from build123d import *

# Parameters (mm, degrees)
F0_W     = 304.8
F0_H     = 297.18
F0_H_2   = 20.32
F1_DEPTH = 17.526
F2_DEPTH = 8.255


with BuildPart() as f1:
    # F0 (on Front) → F1 (new body)
    with BuildSketch(Plane.XZ):
        with Locations((-26.445295, -488.64002)):
            Rectangle(F0_W, F0_H)
        with Locations((-26.445295, -329.89002)):
            Rectangle(F0_W, F0_H_2)
        with BuildLine():
            Line((-178.845295, -299.41002), (-178.845295, -319.73002))
            Line((-178.845295, -319.73002), (125.954705, -319.73002))
            Line((125.954705, -319.73002), (125.954705, -299.41002))
            Line((125.954705, -299.41002), (125.954705, -278.324652))
            Line((125.954705, -278.324652), (125.954705, -258.004652))
            Line((125.954705, -258.004652), (125.954705, 277.16998))
            Line((125.954705, 277.16998), (24.354705, 277.16998))
            Line((24.354705, 277.16998), (24.354705, 226.36998))
            ThreePointArc((24.354705, 226.36998), (-28.678357, -26.576251), (-178.845295, -236.919284))
            Line((-178.845295, -236.919284), (-178.845295, -258.004652))
            Line((-178.845295, -258.004652), (-178.845295, -299.41002))
        make_face()
    extrude(amount=F1_DEPTH)

    # F0 (on Front) → F2 (cut)
    with BuildSketch(Plane.XZ):
        with Locations((-26.445295, -329.89002)):
            Rectangle(F0_W, F0_H_2)
    extrude(amount=F2_DEPTH, mode=Mode.SUBTRACT)


solid = f1.part
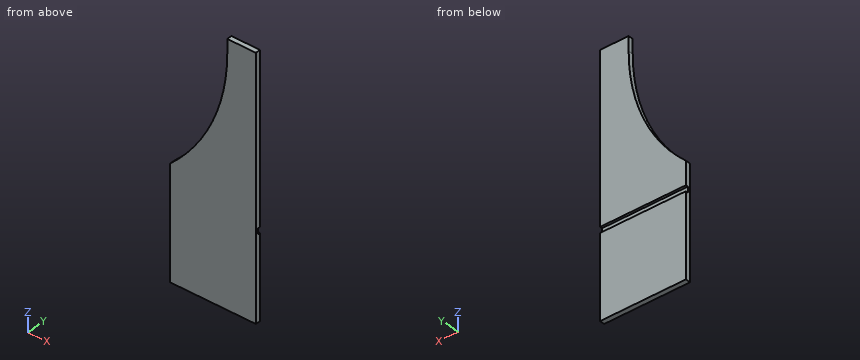
Model file for the job. Use its own axes, mm. Give positions to 0.01 mm unless a question says otherwise; leave off trailing zeros. Order: outer loops, then holes, each group sorted by start corner. A loop starts at its lowest first (then second) coordinate and runs counter-clockwise, first axis right, second up. Notation, with made-up numbers: (20, 45.25) - (53, 45.25) arc R25 cw to (53, 77.25) - close; hole circle Ø7 at (18, 56.25). An arc over 180 degrees is marked (long way). One line per item, written item: value.
Item 1: Slice it at C-C (z = 98). List the corners of the cut face in (x, y), then the cut area to 3 significant figures.
Response values:
outline: (11.13, -17.53) - (125.95, -17.53) - (125.95, 0) - (11.13, 0) - close
area: 2,010 mm2
Item 2: Pin check, flat tips, straight feed: pin 1 Ø4 at (x, y) = (-77.5, -5) entering from +Z; pin 2 Ø9 at (y, z) = (-10.5, 241.5) entering from -X; pin 3 Ø4 at (x, y) = (-54, -2.5) entering from +Z. Stop position of each tip, or through.
Response values:
pin 1: z = -113.92
pin 2: x = 24.35
pin 3: z = -74.19
Item 3: Slice it at D-D (x = -145.5). List the corners of the cut face in (y, z) (3 decimals).
Response values:
outline: (-17.526, -637.23) - (0, -637.23) - (0, -340.05) - (-8.255, -340.05) - (-8.255, -319.73) - (0, -319.73) - (0, -203.838) - (-17.526, -203.838) - close
Item 4: Slice it at B-B (x = -63.5). List the corners of the cut face in (y, z) (3 decimals), then the cut area to 3 significant figures.
Response values:
outline: (-17.526, -637.23) - (0, -637.23) - (0, -340.05) - (-8.255, -340.05) - (-8.255, -319.73) - (0, -319.73) - (0, -94.462) - (-17.526, -94.462) - close
area: 9,340 mm2
Item 5: Slice it at A-A (y = -5). List the corners of the cut face in (x, z).
Response values:
outline: (-178.85, -637.23) - (125.95, -637.23) - (125.95, -340.05) - (-178.85, -340.05) - close; (-178.85, -319.73) - (125.95, -319.73) - (125.95, 277.17) - (24.35, 277.17) - (24.35, 226.37) arc R629.74 cw to (-178.85, -236.92) - close
Item 6: Wall check: line 1 (Z direction, x = 67, y = -7.75); line 2 (Z direction, x = -123.5, y = -16); line 3 (Z direction, x = -115, y = -4.75). Give the ranges that are in metal, low to high.
Response values:
line 1: -637.23 to -340.05, -319.73 to 277.17
line 2: -637.23 to -179.04
line 3: -637.23 to -340.05, -319.73 to -168.72
